```python
from build123d import *

# Parameters (mm, degrees)
SKETCH1_W             = 100
SKETCH1_H             = 94.92
BOSS_EXTRUDE1_DEPTH   = 1.27
SKETCH8_R             = 2.85
SKETCH8_R_2           = 2
BOSS_EXTRUDE3_DEPTH   = 7
M4X0_7_TAPPED_HOLE1_D = 3.3
SKETCH13_R            = 9
SKETCH13_R_2          = 1.1
CUT_EXTRUDE7_DEPTH    = 5
SKETCH14_R            = 1
CUT_EXTRUDE8_DEPTH    = 10
CUT_EXTRUDE9_DEPTH    = 2.54


with BuildPart() as part:
    # Sketch1 → Boss-Extrude1 (new body)
    with BuildSketch(Plane.XY):
        with Locations((50, 48.73)):
            Rectangle(SKETCH1_W, SKETCH1_H)
    extrude(amount=BOSS_EXTRUDE1_DEPTH)

    # Sketch8 → Boss-Extrude3 (add)
    with BuildSketch(Plane(origin=(0, 0, 0), x_dir=(-1, 0, 0), z_dir=(0, 0, -1))):
        with Locations((-81.00001, 73.05481987)):
            Circle(SKETCH8_R)
        with Locations((-81.00001, 73.05481987)):
            Circle(SKETCH8_R_2, mode=Mode.SUBTRACT)
        with Locations((-81.00001, 73.05481987)):
            Circle(SKETCH8_R_2)
        with Locations((-41.00001, 73.05481987)):
            Circle(SKETCH8_R)
        with Locations((-41.00001, 73.05481987)):
            Circle(SKETCH8_R_2, mode=Mode.SUBTRACT)
        with Locations((-41.00001, 73.05481987)):
            Circle(SKETCH8_R_2)
    extrude(amount=-BOSS_EXTRUDE3_DEPTH)

    # M4x0.7 Tapped Hole1 (through all)
    with Locations(Plane.XY.offset(7)):
        with Locations((81.00001, 73.05481987), (41.00001, 73.05481987)):
            Hole(M4X0_7_TAPPED_HOLE1_D / 2)

    # Sketch13 → Cut-Extrude7 (cut)
    with BuildSketch(Plane(origin=(0, 0, 0), x_dir=(-1, 0, 0), z_dir=(0, 0, -1))):
        with Locations((-25.031645402, 15)):
            Circle(SKETCH13_R)
        with Locations((-14.031645402, 15)):
            Circle(SKETCH13_R_2)
        with Locations((-25.031645402, 4)):
            Circle(SKETCH13_R_2)
        with Locations((-36.031645402, 15)):
            Circle(SKETCH13_R_2)
        with Locations((-25.031645402, 26)):
            Circle(SKETCH13_R_2)
    extrude(amount=-CUT_EXTRUDE7_DEPTH, mode=Mode.SUBTRACT)

    # Sketch14 → Cut-Extrude8 (cut)
    with BuildSketch(Plane(origin=(0, 0, 0), x_dir=(-1, 0, 0), z_dir=(0, 0, -1))):
        with Locations(Location((-2.5, 73.73, 0), (0, 0, 180))):
            Circle(SKETCH14_R)
        with Locations(Location((-2.5, 23.73, 0), (0, 0, 180))):
            Circle(SKETCH14_R)
        with Locations((-97.5, 23.73)):
            Circle(SKETCH14_R)
        with Locations((-97.5, 73.73)):
            Circle(SKETCH14_R)
    extrude(amount=-CUT_EXTRUDE8_DEPTH, mode=Mode.SUBTRACT)

    # Sketch15 → Cut-Extrude9 (cut)
    with BuildSketch(Plane.XY.offset(1.27)):
        with BuildLine():
            Line((5.801106051, 51.665736829), (5.801106051, 70.837304612))
            ThreePointArc((5.801106051, 70.837304612), (6.545054826, 72.633355836), (8.341106051, 73.377304612))
            Line((8.341106051, 73.377304612), (11.435588088, 73.377304612))
            ThreePointArc((11.435588088, 73.377304612), (13.231639313, 72.633355836), (13.975588088, 70.837304612))
            Line((13.975588088, 70.837304612), (13.975588088, 51.665736829))
            ThreePointArc((13.975588088, 51.665736829), (13.231639313, 49.869685605), (11.435588088, 49.125736829))
            Line((11.435588088, 49.125736829), (8.341106051, 49.125736829))
            ThreePointArc((8.341106051, 49.125736829), (6.545054826, 49.869685605), (5.801106051, 51.665736829))
        make_face()
    extrude(amount=-CUT_EXTRUDE9_DEPTH, mode=Mode.SUBTRACT)


solid = part.part
```
Build history of the part. All positions in model axes, mm. A direction names the side the tool comes from. Give positions to 0.01 mm unless a question says otherwise; leave off trailing zeros. Loops run counter-clockwise (first coordinate to the right, second up) from the corner with the lowest first, then second, coordinate; pieces in that order, holes last.
1) Band-saw the part on A-A on y = 53. List the corners of the cut face in (x, z).
Values follow:
outline: (0, 0) - (5.8, 0) - (5.8, 1.27) - (0, 1.27) - close; (13.98, 0) - (100, 0) - (100, 1.27) - (13.98, 1.27) - close
2) Band-saw the part on D-D on y = 89. List the corners of the cut face in (x, z).
Values follow:
outline: (0, 0) - (100, 0) - (100, 1.27) - (0, 1.27) - close
3) Probe line 1 along Y through (x, z) = (97.5, 0.5); line 2 along Z through (x, y) = (80, 64); line 3 along Y through (x, z) = (80.5, 6.5). List the from-to ranges inside material, lowest first.
Values follow:
line 1: y = 1.27 to 22.73, 24.73 to 72.73, 74.73 to 96.19
line 2: z = 0 to 1.27
line 3: y = 70.25 to 71.48, 74.63 to 75.86
4) 3-axis set-ups, long thin cutter, end or side, ignore diameter. For faces 3 (the face through (81, 71, 7)), 4 (the face through (6.565, 49.85, 0.644)), 5 (the face through (79.68, 70.53, 4.09)): which of +Z, -Z, +X, -X, +Y, -Y reach the whole face in a straight line?
Values follow:
face 3: +Z, +X, -X, +Y, -Y
face 4: +Z, -Z
face 5: +Z
5) Drop a flat-ended pin along its axis: P1, Ø1.5, axis at x = 61.5, y = 14.5, coming from the +Z side. Give the stop position or say it passes through.
Values follow:
P1: stops at z = 1.27
6) Band-saw the part on B-B on x = 19.5. List the corners of the cut face in (y, z), then the cut area to 3 significant figures.
Values follow:
outline: (1.27, 0) - (7.9, 0) - (7.9, 1.27) - (1.27, 1.27) - close; (22.1, 0) - (96.19, 0) - (96.19, 1.27) - (22.1, 1.27) - close
area: 103 mm2
7) Two-plate mould, pull along X, no slides. Class faces 1 (the face through (41, 71, 7)), 2 (the face through (41.618, 70.273, 4.095)): released by +X, released by -X, zero draft, split by the parting line, or undercut.
Values follow:
face 1: zero draft
face 2: undercut
8) Band-saw the part on C-C on z = 3.75. List the corners of the cut face in (x, y).
Values follow:
outline: circle Ø5.7 at (41, 73.05); circle Ø5.7 at (81, 73.05); hole circle Ø3.3 at (41, 73.05); hole circle Ø3.3 at (81, 73.05)
